Geometry: final body of the model. Coordinates: model frame, mm. Face numbers are marked on the shaded views. Coordinates: 2 decimals unless noted, no trailing zeros. Order: outer loops, then holes, each group sorted by start corner. A loop starts at its lowest first (then second) coordinate and runs counter-clockwise, first axis right, second up. Notation, with made-up numbers: M 18.25,18.25 L 64.25,18.25 A19 ccw 64.25,38.25 Z; hole C 80,-8.75 d11. An arc over 180 degrees is marked long. Use CSV: the item, a comma, the result in double quotes. Start each with the question number.
1. Section query B-B on x = 5. Return the cut outline in (y, z).
2. Material intervals for line 1 (Y direction, x = 0, z = 8); line 2 (Y direction, x = -1.5, z = 18); line 3 (X direction, y = -114, z = 15), sorted ascending.
3. Pull-direction query (Y, two-part tool) for the marked faces 1, 2 and 3; classes: pulls with the +Y half, pulls with the -Y half, needs draft (parallel to the pull), parting line crosses it, or undercut.
4. Section query A-A on y = -114.3. Return the cut outline in (x, z).
5. Section query C-C on z = 27.5. Return the cut outline in (x, y), and give its area (3 significant figures).
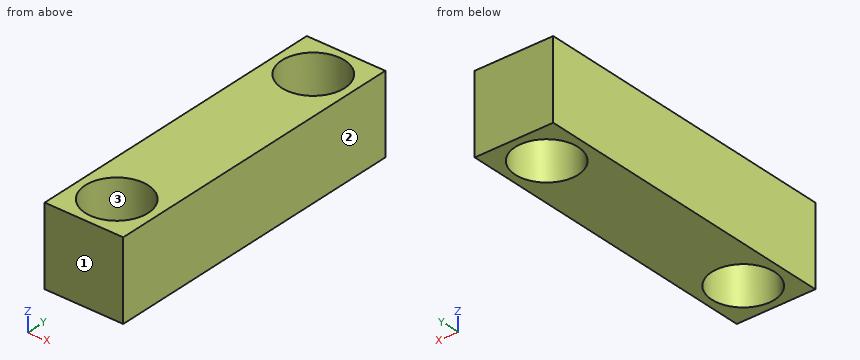
from build123d import *

# Parameters (mm, degrees)
SKETCH1_W           = 25.4
SKETCH1_H           = 101.6
BOSS_EXTRUDE1_DEPTH = 25.4
SKETCH2_R           = 10.16
CUT_EXTRUDE1_DEPTH  = 25.4
SCALE1_SCALE        = 3


with BuildPart() as part:
    # Sketch1 → Boss-Extrude1 (new body)
    with BuildSketch(Plane.XY):
        Rectangle(SKETCH1_W, SKETCH1_H)
    extrude(amount=BOSS_EXTRUDE1_DEPTH)

    # Sketch2 → Cut-Extrude1 (cut)
    with BuildSketch(Plane.XY.offset(25.4)):
        with Locations((0, -38.1)):
            Circle(SKETCH2_R)
        with Locations((0, 38.1)):
            Circle(SKETCH2_R)
    extrude(amount=-CUT_EXTRUDE1_DEPTH, mode=Mode.SUBTRACT)


with BuildPart() as part_1:
    # Scale1: scaled about (0, 0, 12.7)
    add(part.part.scale(SCALE1_SCALE).moved(Location((0, 0, -25.4))))


solid = part_1.part
Results list:
1,outline,"M -152.4,-25.4 L -144.37,-25.4 L -144.37,50.8 L -152.4,50.8 Z; M -84.23,-25.4 L 84.23,-25.4 L 84.23,50.8 L -84.23,50.8 Z; M 144.37,-25.4 L 152.4,-25.4 L 152.4,50.8 L 144.37,50.8 Z"
2,line 1,"y = -152.4 to -144.78, -83.82 to 83.82, 144.78 to 152.4"
2,line 2,"y = -152.4 to -144.74, -83.86 to 83.86, 144.74 to 152.4"
2,line 3,"x = -38.1 to -30.48, 30.48 to 38.1"
3,face 1,"pulls with the -Y half"
3,face 2,"needs draft"
3,face 3,"undercut"
4,outline,"M -38.1,-25.4 L -30.48,-25.4 L -30.48,50.8 L -38.1,50.8 Z; M 30.48,-25.4 L 38.1,-25.4 L 38.1,50.8 L 30.48,50.8 Z"
5,outline,"M -38.1,-152.4 L 38.1,-152.4 L 38.1,152.4 L -38.1,152.4 Z; hole C 0,-114.3 d60.96; hole C 0,114.3 d60.96"
5,area,"17,400 mm²"
